Input: part model. Units: mm. Frame: model coordinates. Face numbers are marked on the shaded views. A direction names the side the tool comes from. Coordinates: 2 decimals unless noted, no trailing zeros. Order: outer loops, then holes, each group sorted by start corner. A loop starts at its lowest first (then second) coordinate and runs counter-clockwise, first axis right, second up. Notation, with made-up numbers: (46, 5.25) -> (74, 5.25) arc R34 ccw to (74, 36.25) -> close; hole circle Ø11 at (-8, -2.5). An arc over 180 degrees is marked (long way). One line per question, with ' | ' between items.
```python
from build123d import *

# Parameters (mm, degrees)
SKETCH1_W           = 110
SKETCH1_H           = 50
SKETCH1_R           = 12.5
BOSS_EXTRUDE1_DEPTH = 10
BOSS_EXTRUDE2_START = 55
SKETCH2_W           = 50
SKETCH2_H           = 65
SKETCH2_R           = 10
BOSS_EXTRUDE2_DEPTH = 10
BOSS_EXTRUDE3_START = -55
SKETCH2_2_W         = 50
SKETCH2_2_H         = 65
SKETCH2_2_R         = 10
BOSS_EXTRUDE3_DEPTH = 10


with BuildPart() as part:
    # Sketch1 → Boss-Extrude1 (new body)
    with BuildSketch(Plane(origin=(0, 0, 0), x_dir=(1, 0, 0), z_dir=(0, 1, 0))):
        Rectangle(SKETCH1_W, SKETCH1_H)
        Circle(SKETCH1_R, mode=Mode.SUBTRACT)
    extrude(amount=BOSS_EXTRUDE1_DEPTH)

    # Sketch2 → Boss-Extrude2 (add)
    with BuildSketch(Plane(origin=(0, 0, 0), x_dir=(0, 0, -1), z_dir=(1, 0, 0)).offset(BOSS_EXTRUDE2_START)):
        with Locations((0, -22.5)):
            Rectangle(SKETCH2_W, SKETCH2_H)
        with Locations((0, -20)):
            Circle(SKETCH2_R, mode=Mode.SUBTRACT)
    extrude(amount=-BOSS_EXTRUDE2_DEPTH)

    # Sketch2<2> → Boss-Extrude3 (add)
    with BuildSketch(Plane(origin=(0, 0, 0), x_dir=(0, 0, -1), z_dir=(1, 0, 0)).offset(BOSS_EXTRUDE3_START)):
        with Locations((0, -22.5)):
            Rectangle(SKETCH2_2_W, SKETCH2_2_H)
        with Locations((0, -20)):
            Circle(SKETCH2_2_R, mode=Mode.SUBTRACT)
    extrude(amount=BOSS_EXTRUDE3_DEPTH)


solid = part.part
```
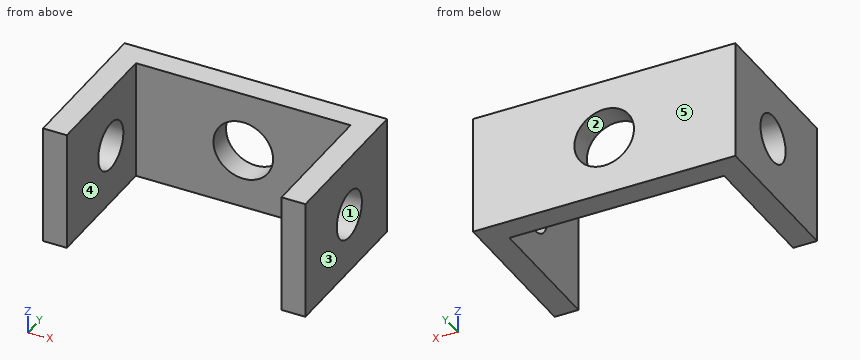
1. Mould query, pull axis X, two halves, no side actions, for the marked faces 1, 2 and 3. Classes: released by +X, released by -X, zero draft, split by the parting line, or undercut.
Recorded:
face 1: zero draft | face 2: undercut | face 3: released by +X
2. Ray query, line 1 (Z direction, x = 0, y = 5); line 2 (X direction, y = -51, z = -18.5); line 3 (X direction, y = 7.5, z = 0). Return the intervals inside material, ascending. Write a range as [from, to].
Recorded:
line 1: z = [-25, -12.5], [12.5, 25] | line 2: x = [-55, -45], [45, 55] | line 3: x = [-55, -12.5], [12.5, 55]
3. Cut plane B-B, the plane z = 0. Return loops of the section in (x, y).
Recorded:
outline: (-55, -55) -> (-45, -55) -> (-45, -30) -> (-55, -30) -> close; (-55, -10) -> (-45, -10) -> (-45, 0) -> (-12.5, 0) -> (-12.5, 10) -> (-55, 10) -> close; (12.5, 0) -> (45, 0) -> (45, -10) -> (55, -10) -> (55, 10) -> (12.5, 10) -> close; (45, -55) -> (55, -55) -> (55, -30) -> (45, -30) -> close
4. Pin query (flat end, axial travel): pin 1 Ø1 at (x, z) = (21.5, -13.5) entering from -Y. Return the tip coordinate at first contact, or that it passes through.
Recorded:
pin 1: stops at y = 0
5. Access query for the marked faces 4 and 5. Directions: +Z, -Z, +X, -X, +Y, -Y. A direction counts if a zero-diameter tool reaches every point of the face in a straight line with its end or side. Return the directions, or none.
Recorded:
face 4: +Z, -Z, -Y | face 5: +Z, -Z, +X, -X, +Y
6. Cut plane D-D, the plane y = -20. Return loops of the section in (x, z), and give its area (3 significant figures).
Recorded:
outline: (-55, -25) -> (-45, -25) -> (-45, -10) -> (-55, -10) -> close; (-55, 10) -> (-45, 10) -> (-45, 25) -> (-55, 25) -> close; (45, -25) -> (55, -25) -> (55, -10) -> (45, -10) -> close; (45, 10) -> (55, 10) -> (55, 25) -> (45, 25) -> close | area: 600 mm^2
7. Cut plane C-C, the plane y = -50. Return loops of the section in (x, z), and give its area (3 significant figures).
Recorded:
outline: (-55, -25) -> (-45, -25) -> (-45, 25) -> (-55, 25) -> close; (45, -25) -> (55, -25) -> (55, 25) -> (45, 25) -> close | area: 1,000 mm^2
8. Cut plane A-A, the plane x = 0.5. Return loops of the section in (y, z).
Recorded:
outline: (0, -25) -> (10, -25) -> (10, -12.49) -> (0, -12.49) -> close; (0, 12.49) -> (10, 12.49) -> (10, 25) -> (0, 25) -> close
